Here's how the part is built. I have some questions about the finished solid (model axes, mm). Round coordinates to 2 decimals unless told otherwise and drop trailing zeros. Order: outer loops, then holes, each group sorted by start corner. A loop starts at its lowest first (then second) coordinate and runs counter-clockwise, first axis right, second up. Notation, with made-up numbers: M 76.25,61 L 87.25,61 A11 ccw 87.25,68 Z; hole C 67.25,-25.5 d1. An arc over 180 degrees is marked long. Use one line per item in the form item = value. Start each with the question number.
```python
from build123d import *

# Parameters (mm, degrees)
EXTRUDE_837_DEPTH      = 5
SKETCH_2_R             = 1.5
CUT_EXTRUDE_1413_DEPTH = 6
FILLET_1486_R          = 10
SKETCH_9_R             = 1.5
CUT_EXTRUDE_2145_DEPTH = 5
SKETCH_35_R            = 1.5
CUT_EXTRUDE_2803_DEPTH = 5
SKETCH_38_R            = 1.5
CUT_EXTRUDE_1_DEPTH    = 5
SKETCH_39_R            = 1.5
CUT_EXTRUDE_2_DEPTH    = 5
SKETCH_40_R            = 1.5
CUT_EXTRUDE_4396_DEPTH = 5
SKETCH_41_R            = 1.5
CUT_EXTRUDE_4966_DEPTH = 5
SKETCH_43_R            = 1.5
CUT_EXTRUDE_5573_DEPTH = 5
SKETCH_44_R            = 1.5
CPU_DEPTH              = 5


with BuildPart() as part:
    # ｽｹｯﾁ1 → Extrude 837 (new body)
    with BuildSketch(Plane(origin=(0, 0, 0), x_dir=(1, 0, 0), z_dir=(0, 1, 0))):
        Polygon((135, -60), (55, 125), (-55, 125), (-135, -60), (-135, -125), (135, -125), align=None)
    extrude(amount=EXTRUDE_837_DEPTH)

    # ｽｹｯﾁ2 → Cut-Extrude 1413 (cut, through all)
    with BuildSketch(Plane.XZ):
        with Locations(Location((-130, 72, 0), (0, 0, 270))):  # turned: the seam where the file's is
            Circle(SKETCH_2_R)
        with Locations(Location((-130, 108, 0), (0, 0, 270))):  # turned: the seam where the file's is
            Circle(SKETCH_2_R)
        with Locations(Location((130, 72, 0), (0, 0, 270))):  # turned: the seam where the file's is
            Circle(SKETCH_2_R)
        with Locations(Location((130, 108, 0), (0, 0, 270))):  # turned: the seam where the file's is
            Circle(SKETCH_2_R)
    extrude(amount=-CUT_EXTRUDE_1413_DEPTH, mode=Mode.SUBTRACT)

    # Fillet 1486
    fillet_1486_edges = [part.edges().sort_by_distance(p)[0] for p in [
        (55, 2.5, -125),
        (135, 2.5, 60),
        (135, 2.5, 125),
        (-135, 2.5, 125),
        (-135, 2.5, 60),
        (-55, 2.5, -125),
    ]]
    fillet(fillet_1486_edges, radius=FILLET_1486_R)

    # ｽｹｯﾁ9 → Cut-Extrude 2145 (cut)
    with BuildSketch(Plane.XZ):
        with Locations(Location((15, -105, 0), (0, 0, 270))):  # turned: the seam where the file's is
            Circle(SKETCH_9_R)
        with Locations(Location((-15, -105, 0), (0, 0, 270))):  # turned: the seam where the file's is
            Circle(SKETCH_9_R)
    extrude(amount=-CUT_EXTRUDE_2145_DEPTH, mode=Mode.SUBTRACT)

    # ｽｹｯﾁ35 → Cut-Extrude 2803 (cut)
    with BuildSketch(Plane.XZ):
        with Locations(Location((-15, 21.5, 0), (0, 0, 270))):  # turned: the seam where the file's is
            Circle(SKETCH_35_R)
        with Locations(Location((15, 21.5, 0), (0, 0, 270))):  # turned: the seam where the file's is
            Circle(SKETCH_35_R)
    extrude(amount=-CUT_EXTRUDE_2803_DEPTH, mode=Mode.SUBTRACT)

    # ｽｹｯﾁ38 → 内側モータマウンタ穴1 (cut)
    with BuildSketch(Plane.XZ):
        with Locations(Location((-100, 72, 0), (0, 0, 270))):  # turned: the seam where the file's is
            Circle(SKETCH_38_R)
        with Locations(Location((-100, 108, 0), (0, 0, 270))):  # turned: the seam where the file's is
            Circle(SKETCH_38_R)
    extrude(amount=-CUT_EXTRUDE_1_DEPTH, mode=Mode.SUBTRACT)

    # ｽｹｯﾁ39 → 内側モータマウンタ穴2 (cut)
    with BuildSketch(Plane(origin=(0, 0, 0), x_dir=(-1, 0, 0), z_dir=(0, -1, 0))):
        with Locations(Location((-100, -72, 0), (0, 0, 90))):  # turned: the seam where the file's is
            Circle(SKETCH_39_R)
        with Locations(Location((-100, -108, 0), (0, 0, 90))):  # turned: the seam where the file's is
            Circle(SKETCH_39_R)
    extrude(amount=-CUT_EXTRUDE_2_DEPTH, mode=Mode.SUBTRACT)

    # ｽｹｯﾁ40 → Cut-Extrude 4396 (cut)
    with BuildSketch(Plane.XZ):
        with Locations(Location((51, -117.5, 0), (0, 0, 270))):  # turned: the seam where the file's is
            Circle(SKETCH_40_R)
        with Locations(Location((-51, -117.5, 0), (0, 0, 270))):  # turned: the seam where the file's is
            Circle(SKETCH_40_R)
        with Locations(Location((51, -102.5, 0), (0, 0, 270))):  # turned: the seam where the file's is
            Circle(SKETCH_40_R)
        with Locations(Location((-51, -102.5, 0), (0, 0, 270))):  # turned: the seam where the file's is
            Circle(SKETCH_40_R)
    extrude(amount=-CUT_EXTRUDE_4396_DEPTH, mode=Mode.SUBTRACT)

    # ｽｹｯﾁ41 → Cut-Extrude 4966 (cut)
    with BuildSketch(Plane.XZ):
        with Locations(Location((75, 15, 0), (0, 0, 270))):  # turned: the seam where the file's is
            Circle(SKETCH_41_R)
        with Locations(Location((75, -10, 0), (0, 0, 270))):  # turned: the seam where the file's is
            Circle(SKETCH_41_R)
        with Locations(Location((-75, 15, 0), (0, 0, 270))):  # turned: the seam where the file's is
            Circle(SKETCH_41_R)
        with Locations(Location((-75, -10, 0), (0, 0, 270))):  # turned: the seam where the file's is
            Circle(SKETCH_41_R)
    extrude(amount=-CUT_EXTRUDE_4966_DEPTH, mode=Mode.SUBTRACT)

    # ｽｹｯﾁ43 → Cut-Extrude 5573 (cut)
    with BuildSketch(Plane.XZ):
        with Locations(Location((-55, 0, 0), (0, 0, 270))):  # turned: the seam where the file's is
            Circle(SKETCH_43_R)
        with Locations(Location((-55, -66, 0), (0, 0, 270))):  # turned: the seam where the file's is
            Circle(SKETCH_43_R)
        with Locations(Location((55, 0, 0), (0, 0, 270))):  # turned: the seam where the file's is
            Circle(SKETCH_43_R)
        with Locations(Location((55, -66, 0), (0, 0, 270))):  # turned: the seam where the file's is
            Circle(SKETCH_43_R)
    extrude(amount=-CUT_EXTRUDE_5573_DEPTH, mode=Mode.SUBTRACT)

    # ｽｹｯﾁ44 → CPUタワー穴 (cut)
    with BuildSketch(Plane.XZ):
        with Locations(Location((-41, 32, 0), (0, 0, 270))):  # turned: the seam where the file's is
            Circle(SKETCH_44_R)
        with Locations(Location((40, 32, 0), (0, 0, 270))):  # turned: the seam where the file's is
            Circle(SKETCH_44_R)
        with Locations(Location((38, 117, 0), (0, 0, 270))):  # turned: the seam where the file's is
            Circle(SKETCH_44_R)
        with Locations(Location((-37, 117, 0), (0, 0, 270))):  # turned: the seam where the file's is
            Circle(SKETCH_44_R)
    extrude(amount=-CPU_DEPTH, mode=Mode.SUBTRACT)


solid = part.part
```
1) If I drill on line 1 (X direction, y = 2.3, z = 15); line 2 (X direction, y = 1.85, z = -66); line 3 (X direction, y = 1.2, z = 107.5), over which ranges is the centre line in solid material (lowest first)?
2) If we section it at B-B on x = -65.5: Write out the boundary of the cut face in (y, z), then the cut area to 3 significant figures.
3) If we section it at A-A on y = 2: Give the number of separate pieces and of enclosed holes in the cut face, then the cut area to 3 significant figures.
4) Will these pins go through, and if not, where does the flat tip stop? pin 1 Ø2 at (y, z) = (1.5, 36) entering from -X; pin 2 Ø1 at (y, z) = (2, 20) entering from +X.
Completed:
q1.line_1 = -115.54 to -76.5, -73.5 to 73.5, 76.5 to 115.54
q1.line_2 = -80.51 to -56.5, -53.5 to 53.5, 56.5 to 80.51
q1.line_3 = -135 to -131.41, -128.59 to -101.41, -98.59 to 98.59, 101.41 to 128.59, 131.41 to 135
q2.outline = M 0,-100.72 L 5,-100.72 L 5,125 L 0,125 Z
q2.area = 1,130 mm²
q3.separate_pieces = 1
q3.enclosed_holes = 28
q3.area = 52,400 mm²
q4.pin_1 = -125.05
q4.pin_2 = 117.92
